Design review of the part shown in the three views and the two pictorial views. Dimensions are in mm from the part's minimum x, y and z. Round coordinates to 2 decimals unless told otherwise and drop trailing zeros. Write each loop counter-clockwise with the first axis right and the second up, starting at its lowest first coordinate (ties: lowest second). Pieces come first, ordered by that corner, then holes. Notation, with made-up numbers: (-26, 55) -> (19, 55) arc R27 cw to (19, 82) -> close; hole circle Ø11 at (-35, 74.25). An arc over 180 degrees is marked (long way). Answer as a JSON object with one key per item and string values. Group by question number.
1) To check wall thickness, follow probe 1 along Y at (x, z) = (3, 36.5); probe 2 along Y at (x, z) = (2.05, 24.5); probe 3 along X at (y, z) = (3.25, 4.5). State the ranges of each line that lie inside material, in increasing order. Write a range as [from, to].
2) Insertion check: pin 1 Ø1.5 at (x, y) = (3, 3) entering from +Z; pin 2 Ø1 at (y, z) = (5, 16.5) entering from -X; pin 3 Ø2 at (y, z) = (1.5, 41) entering from +X. Each pin has a flat end and moves straight along its axis. Give the tip position at first contact, or say it passes through.
3) We need section C-C, the plane z = 31.5. Write out the cut boundary in (x, y), then the cut area to 3 significant figures.
4) We need section D-D, the plane x = 5.2. Write out the cut boundary in (y, z), then the cut area to 3 significant figures.
5) We need section B-B, the plane x = 2.15. Write out the cut boundary in (y, z), then the cut area to 3 significant figures.
6) We need section A-A, the plane y = 3. Write out the cut boundary in (x, z).
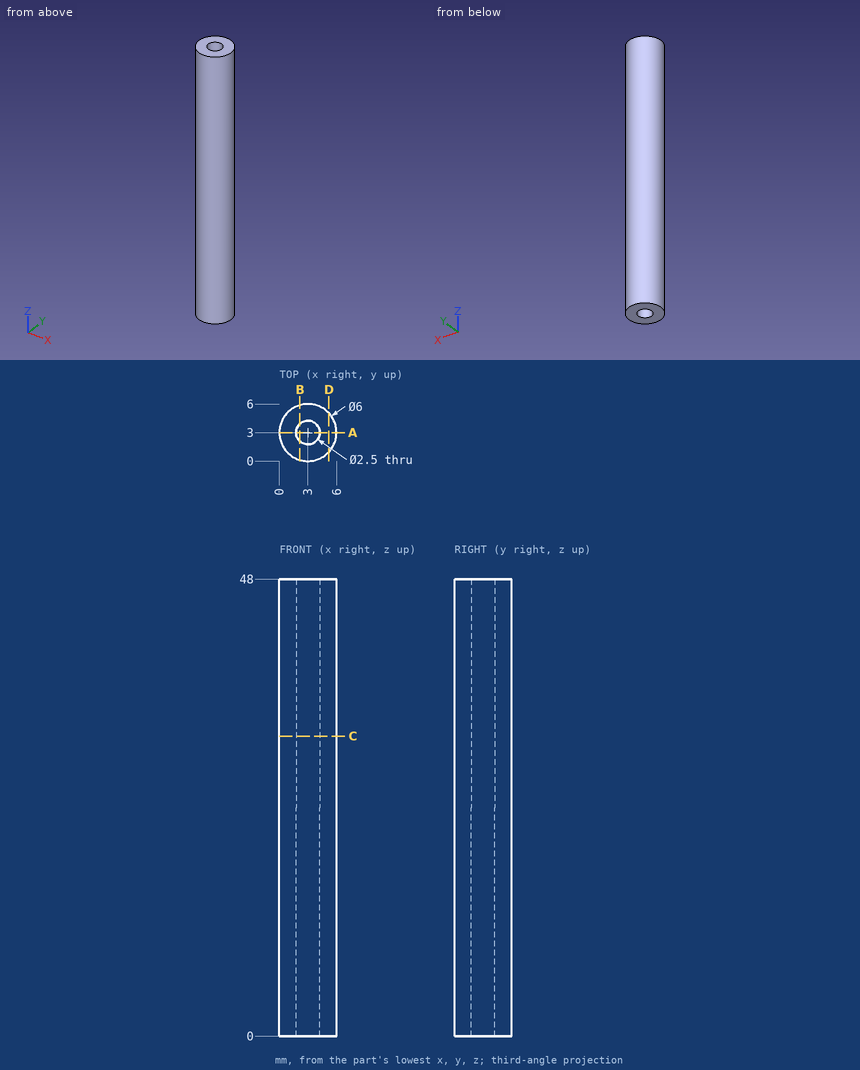
Here are the results:
{
 "1": {"probe 1": "y = [0, 1.75], [4.25, 6]", "probe 2": "y = [0.15, 2.19], [3.81, 5.85]", "probe 3": "x = [0.01, 1.78], [4.22, 5.99]"},
 "2": {"pin 1": "passes through", "pin 2": "stops at x = 0.4", "pin 3": "stops at x = 5.96"},
 "3": {"outline": "circle Ø6 at (3, 3); hole circle Ø2.5 at (3, 3)", "area": "23.4 mm^2"},
 "4": {"outline": "(0.96, 0) -> (5.04, 0) -> (5.04, 48) -> (0.96, 48) -> close", "area": "196 mm^2"},
 "5": {"outline": "(0.12, 0) -> (2.08, 0) -> (2.08, 48) -> (0.12, 48) -> close; (3.92, 0) -> (5.88, 0) -> (5.88, 48) -> (3.92, 48) -> close", "area": "188 mm^2"},
 "6": {"outline": "(0, 0) -> (1.75, 0) -> (1.75, 48) -> (0, 48) -> close; (4.25, 0) -> (6, 0) -> (6, 48) -> (4.25, 48) -> close"}
}
